from build123d import *

# Parameters (mm, degrees)
F3_D    = 26.19502
F4_R    = 3
F5_SIZE = 5
F6_SIZE = 5


with BuildPart() as f1:
    # F0 (on Front) → F1 (revolve)
    with BuildSketch(Plane.XZ):
        Polygon((21.85, 109.5), (21.85, 0), (41.672, 0), (45.0412688537, 7.9375), (50.2088311463, 7.9375), (53.5781, 0), (62.0001, 0), (62.0001, 8), (107.5, 8), (107.5, 46.1), (52.4, 46.1), (30.15, 97.1311859998), (30.15, 103.1311859998), align=None)
    revolve(axis=Axis((0, 0, 78.9197534323), (0, 0, 1)))

    # F3 (through all)
    with Locations(Plane.XY.offset(46.1)):
        with Locations((0, 82.55), (58.3716647869, 58.3716647869), (82.55, 0), (58.3716647869, -58.3716647869), (0, -82.55), (-58.3716647869, -58.3716647869), (-82.55, 0), (-58.3716647869, 58.3716647869)):
            Hole(F3_D / 2)

    # F4
    f4_edges = [f1.edges().sort_by_distance(p)[0] for p in [
        (-52.4, 0, 46.1),
    ]]
    fillet(f4_edges, radius=F4_R)

    # F5
    f5_edges = [f1.edges().sort_by_distance(p)[0] for p in [
        (-107.5, 0, 8),
    ]]
    chamfer(f5_edges, length=F5_SIZE)

    # F6
    f6_edges = [f1.edges().sort_by_distance(p)[0] for p in [
        (-107.5, 0, 46.1),
    ]]
    chamfer(f6_edges, length=F6_SIZE)


solid = f1.part
Build history of the part. All positions in model axes, mm. A direction names the side the tool comes from. Round coordinates to 2 decimals unless told otherwise and drop trailing zeros. Write each loop counter-clockwise with the first axis right and the second up, starting at its lowest first coordinate (ties: lowest second). Pieces come first, ordered by that corner, then holes. Notation, with made-up numbers: (-34.5, -24) - (3.5, -24) arc R14 ccw to (3.5, -10) - close; hole circle Ø3 at (-13.5, -29). An arc over 180 degrees is marked (long way). One line per question, with ' | ' between items.
1. Drill centre lines: line 1 along Y through (x, z) = (7, 22); line 2 along X through (y, z) = (82, 16); line 3 along X through (y, z) = (69, 13.5). Where is each one in solid material? Low to high. Write a range as from..to.
Results are:
line 1: -107.27..-93.62, -71.48..-20.7, 20.7..71.48, 93.62..107.27 | line 2: -69.51..-13.09, 13.09..69.51 | line 3: -82.43..-66.03, -50.72..50.72, 66.03..82.43
2. Mould opens along Y. For faces 1 (the face through (-6.536, -29.433, 100.173)), 2 (the face through (-95.043, 3.934, 26.783)), 3 (the face through (51, -18, 0)) say: released by +Y, released by -Y, zero draft, split by the parting line, or undercut.
Results are:
face 1: split by the parting line | face 2: undercut | face 3: zero draft
3. Drop flat-ended pins along their axis: pin 1 Ø3 at (x, y) = (62.5, -48) entering from +Z; pin 2 Ø1 at (x, y) = (-80, -38) entering from +Z; pin 3 Ø1 at (y, z) = (20.5, 15.5) entering from -X; pin 4 Ø12 at (x, z) = (46, 22) entering from -Y. Give the stop position or say it passes through.
Results are:
pin 1: through | pin 2: z = 46.1 | pin 3: x = -105.62 | pin 4: y = -99.78
4. Band-saw the part on D-D, the plane z = 72.5. Write the cut outline in (x, y).
Results are:
outline: circle Ø81.78 at (0, 0); hole circle Ø43.7 at (0, 0)
5. Band-saw the part on A-A, the plane z = 100. Write the cut outline in (x, y), and give its area (3 significant figures).
Results are:
outline: circle Ø60.3 at (0, 0); hole circle Ø43.7 at (0, 0) | area: 1,360 mm^2
6. Tool access for faces 4 (the face through (44, -44, 46.1)), 5 (the face through (-61.94, 2.73, 4.06)), 6 (the face through (-18, -18, 0)): list every direction of +Z, -Z, +X, -X, +Y, -Y with a clear straight run to the whole face (end or side of a thin tool).
Results are:
face 4: +Z | face 5: -Z | face 6: -Z, +X, -X, +Y, -Y
7. Band-saw the part on B-B, the plane x = 0. Give the number of separate pieces and of enclosed holes in the cut face, and give its area (3 significant figures).
Results are:
separate pieces: 4 | enclosed holes: 0 | area: 7,120 mm^2
